```python
from build123d import *

# Parameters (mm, degrees)
SKETCH1_W           = 600
SKETCH1_H           = 5
BOSS_EXTRUDE1_DEPTH = 100
SKETCH5_W           = 600
SKETCH5_H           = 10
CUT_EXTRUDE1_DEPTH  = 3
SKETCH6_R           = 2
CUT_EXTRUDE2_DEPTH  = 6
SKETCH7_R           = 3
CUT_EXTRUDE3_DEPTH  = 6


with BuildPart() as part:
    # Sketch1 → Boss-Extrude1 (new body)
    with BuildSketch(Plane.XY):
        with Locations((300, 2.5)):
            Rectangle(SKETCH1_W, SKETCH1_H)
    extrude(amount=-BOSS_EXTRUDE1_DEPTH)

    # Sketch5 → Cut-Extrude1 (cut)
    with BuildSketch(Plane(origin=(0, 5, 0), x_dir=(1, 0, 0), z_dir=(0, 1, 0))):
        with Locations((300, 85)):
            Rectangle(SKETCH5_W, SKETCH5_H)
        with Locations((300, 15)):
            Rectangle(SKETCH5_W, SKETCH5_H)
    extrude(amount=-CUT_EXTRUDE1_DEPTH, mode=Mode.SUBTRACT)

    # Sketch6 → Cut-Extrude2 (cut, through all)
    with BuildSketch(Plane(origin=(0, 5, 0), x_dir=(1, 0, 0), z_dir=(0, 1, 0))):
        with Locations((62, 85)):
            Circle(SKETCH6_R)
        with Locations((62, 15)):
            Circle(SKETCH6_R)
        with Locations((538, 85)):
            Circle(SKETCH6_R)
        with Locations((538, 15)):
            Circle(SKETCH6_R)
    extrude(amount=-CUT_EXTRUDE2_DEPTH, mode=Mode.SUBTRACT)

    # Sketch7 → Cut-Extrude3 (cut, through all)
    with BuildSketch(Plane(origin=(0, 5, 0), x_dir=(1, 0, 0), z_dir=(0, 1, 0))):
        with Locations((75, 85)):
            Circle(SKETCH7_R)
        with Locations((75, 15)):
            Circle(SKETCH7_R)
        with Locations((525, 85)):
            Circle(SKETCH7_R)
        with Locations((525, 15)):
            Circle(SKETCH7_R)
    extrude(amount=-CUT_EXTRUDE3_DEPTH, mode=Mode.SUBTRACT)


solid = part.part
```
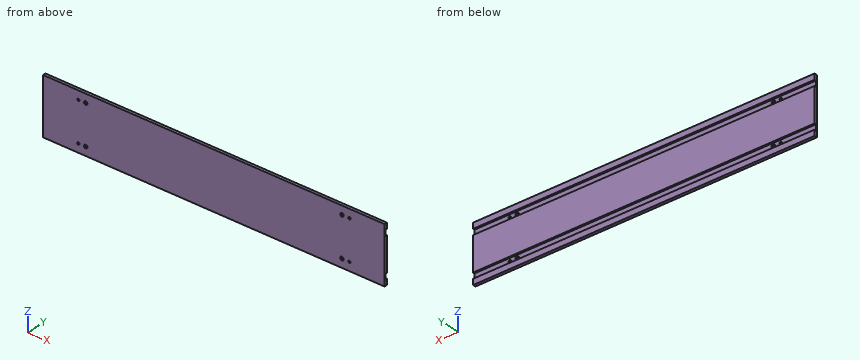
For this review, take the finished solid that the model builds, in its own axes (mm). Round coordinates to 2 decimals unless told otherwise and drop trailing zeros. Write each loop counter-clockwise with the first axis right and the second up, starting at its lowest first coordinate (ties: lowest second). Pieces come first, ordered by that corner, then holes. Notation, with made-up numbers: (79.25, -36.5) - (118.25, -36.5) arc R30 cw to (118.25, -7.5) - close; hole circle Ø5 at (58.5, 63). An arc over 180 degrees is marked (long way). Answer as a JSON object with one key per item and string values.
1. For pin 1 Ø3 at (x, z) = (362.5, -17) entering from +Y, flat-tipped, find the tip position at first contact; note if it passes through.
Response values:
{"pin 1": "stops at y = 2"}
2. We need section A-A on x = 53. Give the boundary of the cut face in (y, z), then the cut area to 3 significant figures.
Response values:
{"outline": "(0, -100) - (5, -100) - (5, -90) - (2, -90) - (2, -80) - (5, -80) - (5, -20) - (2, -20) - (2, -10) - (5, -10) - (5, 0) - (0, 0) - close", "area": "440 mm2"}
3. To check wall thickness, follow line 1 along Z through (x, y) = (62, 1.3); line 2 along Z through (x, y) = (114, 3.1); line 3 along X through (y, z) = (0.55, -15). State the ranges of each line that lie inside material, in increasing order.
Response values:
{"line 1": "z = -100 to -87, -83 to -17, -13 to 0", "line 2": "z = -100 to -90, -80 to -20, -10 to 0", "line 3": "x = 0 to 60, 64 to 72, 78 to 522, 528 to 536, 540 to 600"}
